```python
from build123d import *

# Parameters (mm, degrees)
EXTRUDE_1_DEPTH     = 4
EXTRUDE_2_DEPTH     = 10.5
SKETCH_3_W          = 4.5
SKETCH_3_H          = 4.5
EXTRUDE_3_DEPTH     = 2.5
SKETCH_6_W          = 5.635445318
SKETCH_6_H          = 5.939696962
CUT_EXTRUDE_2_DEPTH = 2.5


with BuildPart() as part:
    # 草图1 → 凸台-拉伸1 (new body)
    with BuildSketch(Plane(origin=(0, 0, 0), x_dir=(1, 0, 0), z_dir=(0, 1, 0))):
        Polygon((2.189696962, -3.75), (3.75, -2.189696962), (3.75, 2.189696962), (2.189696962, 3.75), (-2.189696962, 3.75), (-3.75, 2.189696962), (-3.75, -2.189696962), (-2.189696962, -3.75), align=None)
        with BuildLine():
            Line((2.25, -0.4), (2.25, -2.25))
            Line((2.25, -2.25), (0.4, -2.25))
            ThreePointArc((0.4, -2.25), (0, -2.65), (-0.4, -2.25))
            Line((-0.4, -2.25), (-2.25, -2.25))
            Line((-2.25, -2.25), (-2.25, -0.4))
            ThreePointArc((-2.25, -0.4), (-2.65, 0), (-2.25, 0.4))
            Line((-2.25, 0.4), (-2.25, 2.25))
            Line((-2.25, 2.25), (-0.4, 2.25))
            ThreePointArc((-0.4, 2.25), (0, 2.65), (0.4, 2.25))
            Line((0.4, 2.25), (2.25, 2.25))
            Line((2.25, 2.25), (2.25, 0.4))
            ThreePointArc((2.25, 0.4), (2.65, 0), (2.25, -0.4))
        make_face(mode=Mode.SUBTRACT)
    extrude(amount=EXTRUDE_1_DEPTH)

    # 草图2 → 凸台-拉伸2 (add)
    with BuildSketch(Plane(origin=(0, 4, 0), x_dir=(1, 0, 0), z_dir=(0, 1, 0))):
        Polygon((-2.189696962, -3.75), (2.189696962, -3.75), (3.75, -2.189696962), (3.75, 2.189696962), (2.189696962, 3.75), (-2.189696962, 3.75), (-3.75, 2.189696962), (-3.75, -2.189696962), align=None)
    extrude(amount=EXTRUDE_2_DEPTH)

    # 草图3 → 凸台-拉伸3 (add)
    with BuildSketch(Plane(origin=(0, 14.5, 0), x_dir=(1, 0, 0), z_dir=(0, 1, 0))):
        Rectangle(SKETCH_3_W, SKETCH_3_H)
    extrude(amount=EXTRUDE_3_DEPTH)

    # 草图4 → 旋转1 (revolve)
    with BuildSketch(Plane(origin=(0, 17, 0), x_dir=(1, 0, 0), z_dir=(0, 1, 0))):
        with BuildLine():
            Line((0, 2.75), (0, 1.75))
            ThreePointArc((0, 1.75), (-0.5, 2.25), (0, 2.75))
        make_face()
        with BuildLine():
            Line((0, -1.75), (0, -2.75))
            ThreePointArc((0, -2.75), (-0.5, -2.25), (0, -1.75))
        make_face()
    revolve(axis=Axis((0, 17, -2.75), (0, 0, 1)))

    # 草图5 → 旋转2 (revolve)
    with BuildSketch(Plane(origin=(0, 17, 0), x_dir=(1, 0, 0), z_dir=(0, 1, 0))):
        with BuildLine():
            Line((-2.75, 0), (-1.75, 0))
            ThreePointArc((-1.75, 0), (-2.25, -0.5), (-2.75, 0))
        make_face()
        with BuildLine():
            Line((1.75, 0), (2.75, 0))
            ThreePointArc((2.75, 0), (2.25, -0.5), (1.75, 0))
        make_face()
    revolve(axis=Axis((-2.75, 17, 0), (1, 0, 0)))

    # 草图6 → 切除-拉伸2 (cut)
    with BuildSketch(Plane(origin=(0, 17, 0), x_dir=(1, 0, 0), z_dir=(0, 1, 0))):
        Rectangle(SKETCH_6_W, SKETCH_6_H)
    extrude(amount=CUT_EXTRUDE_2_DEPTH, mode=Mode.SUBTRACT)


solid = part.part
```
Input: part model. Units: mm. Frame: model coordinates. A direction names the side the tool comes from. Round coordinates to 2 decimals unless told otherwise and drop trailing zeros. Order: outer loops, then holes, each group sorted by start corner. A loop starts at its lowest first (then second) coordinate and runs counter-clockwise, first axis right, second up. Notation, with made-up numbers: (-37, 6.25) - (19, 6.25) arc R24 ccw to (19, 45.25) - close; hole circle Ø3 at (-24.75, -14.75). An arc over 180 degrees is marked (long way). One line per question, with ' | ' between items. Start each with the question number.
1) Cut plane D-D, the plane z = 0. Return the cut outline in (x, y), then the cut area to 3 significant figures.
2) Ray query, probe 1 along Y at (x, z) = (-1.25, 0.5); probe 2 along X at (y, z) = (3.25, -1.5); probe 3 along Y at (x, z) = (0.75, 2.5). Return the intervals inside material, ascending.
3) Set-up query: faces 1 (the flat face through (-2.98, 7.15, 2.96)), 2 (the flat face through (-2.25, 2, 1)). Return all of +Z, -Z, +X, -X, +Y, -Y with unobstructed straight access to the full face (end or side cutting, diameter ignored); none if empty.
4) Contact query for flat-ended pins moving along their axis: P1, Ø1.2, axis at x = -0.5, y = 15.5, coming from the +Z side; P2, Ø2, axis at y = 16.5, z = 1, coming from the +X side; P3, Ø0.8, axis at y = 16, z = 0, coming from the -X side. Output: stop coordinate, or through.
5) Cut plane A-A, the plane z = 1.75. Return the cut outline in (x, y), then the cut area to 3 significant figures.
6) Cut plane C-C, the plane y = 12. Return the cut outline in (x, z), then the cut area to 3 significant figures.
7) Pull-direction query (Z, two-part tool) for faces 3 (the flat face through (-1, 0, -3)), 4 (the flat face through (-1, 2, 2.25)), 5 (the flat face through (0, 16, 2.25)); classes: +Z half, -Z half, draft (parallel to the pull), parting line (faces both ways), or undercut.
8) Cut plane B-B, the plane x = 0. Return the cut outline in (y, z).
Worked out:
1) outline: (-3.75, 0) - (-2.65, 0) - (-2.65, 4) - (2.65, 4) - (2.65, 0) - (3.75, 0) - (3.75, 14.5) - (2.25, 14.5) - (2.25, 16.5) arc R0.5 ccw to (2.75, 17) - (-2.75, 17) arc R0.5 ccw to (-2.25, 16.5) - (-2.25, 14.5) - (-3.75, 14.5) - close | area: 99.2 mm^2
2) probe 1: y = 4 to 17 | probe 2: x = -3.75 to -2.25, 2.25 to 3.75 | probe 3: y = 0 to 14.5
3) face 1: +Z, -X, +Y, -Y | face 2: -Y
4) P1: stops at z = 2.25 | P2: stops at x = 2.74 | P3: stops at x = -2.25
5) outline: (-3.75, 0) - (-2.25, 0) - (-2.25, 4) - (2.25, 4) - (2.25, 0) - (3.75, 0) - (3.75, 14.5) - (2.25, 14.5) - (2.25, 17) - (-2.25, 17) - (-2.25, 14.5) - (-3.75, 14.5) - close | area: 102 mm^2
6) outline: (-3.75, -2.19) - (-2.19, -3.75) - (2.19, -3.75) - (3.75, -2.19) - (3.75, 2.19) - (2.19, 3.75) - (-2.19, 3.75) - (-3.75, 2.19) - close | area: 51.4 mm^2
7) face 3: draft | face 4: undercut | face 5: +Z half
8) outline: (0, -3.75) - (14.5, -3.75) - (14.5, -2.25) - (16.5, -2.25) arc R0.5 ccw to (17, -2.75) - (17, 2.75) arc R0.5 ccw to (16.5, 2.25) - (14.5, 2.25) - (14.5, 3.75) - (0, 3.75) - (0, 2.65) - (4, 2.65) - (4, -2.65) - (0, -2.65) - close
